Geometry: final body of the model. Coordinates: model frame, mm. Face numbers are marked on the shaded views. A direction names the side the tool comes from. Give positions to 0.01 mm unless a question says otherwise; leave off trailing zeros. Write each loop counter-clockwise with the first axis right and the second up, starting at its lowest first coordinate (ties: lowest second). Pieces come first, ordered by that corner, then holes. Notation, with made-up numbers: (-32, 50.5) -> (26, 50.5) arc R19 ccw to (26, 74.5) -> close; hole circle Ø4 at (68, 87). An arc over 180 degrees is marked (long way). Answer in a Markdown table with one row per item. Add a question column.
Item 1: Material intervals for probe 1 along Z at (x, y) = (61.5, 4.3); probe 2 along Z at (x, y) = (16, 7.8); probe 3 along X at (y, z) = (7.85, 12.5), sorted ascending. Write a range as from..to.
Item 2: Access query for the marked faces 1, 2 and 3. Directions: +Z, -Z, +X, -X, +Y, -Y. A direction counts if a zero-diameter tool reaches every point of the face in a straight line with its end or side. Return the directions, or none.
Item 3: Section query D-D on x = 61.5. State how many separate pieces and enclosed holes the cut face has, plus the area to 3 significant figures.
Item 4: Section query C-C on z = -4. Output: boundary loops of the cut face in (x, y).
Item 5: First-contact query: P1, Ø2.5, axis at x = 61.5, z = 4, coming from the +Y side; P2, Ø1.8, axis at x = 61.5, z = -4, coming from the +Y side; P3, Ø6, axis at y = 2.5, z = -12, coming from the +X side; P4, Ø3, axis at x = 45, y = 5, coming from the +Z side. Flat tips, straight axial feed; report the tip coordinate or a pass-through.
Item 6: Section query A-A on x = 16. Output: boundary loops of the cut face in (y, z), plus the area to 3 significant figures.
Item 7: Section query B-B on y = 8.75. Output: boundary loops of the cut face in (x, z), plus the area to 3 significant figures.
Autodesk Inventor part; units mm, degrees
ref_plane "YZ Plane" through (0, 0, 0) normal (1, 0, 0) x (0, 1, 0)
ref_plane "XZ Plane" through (0, 0, 0) normal (0, 1, 0) x (-1, 0, 0)
ref_plane "XY Plane" through (0, 0, 0) normal (0, 0, 1) x (1, 0, 0)
sketch "Sketch1" plane through (0, 0, 0) normal (0, 1, 0) x (-1, 0, 0)
  line L0 (-16, 12.5) -> (16, 12.5) construction
  line L1 (16, 12.5) -> (16, -12.5) construction
  line L2 (16, -12.5) -> (-16, -12.5) construction
  line L3 (-16, -12.5) -> (-16, 12.5) construction
  line L4 (-16, 12.5) -> (16, -12.5) construction
  line L5 (16, 12.5) -> (-16, -12.5) construction
  circle A0 centre (16, 12.5) radius 1.65
  circle A1 centre (16, -12.5) radius 1.65
  circle A2 centre (-16, -12.5) radius 1.65
  circle A3 centre (-16, 12.5) radius 1.65
  line L6 (-25, 17) -> (25, 17)
  line L7 (25, 17) -> (25, -17)
  line L8 (25, -17) -> (-25, -17)
  line L9 (-25, -17) -> (-25, 17)
  line L10 (-25, 17) -> (25, -17) construction
  line L11 (25, 17) -> (-25, -17) construction
  point P0 (0, 0)
  dimension "d0" = 32
  dimension "d1" = 25
  dimension "d2" = 3.3
  dimension "d3" = 3.3
  dimension "d4" = 3.3
  dimension "d5" = 3.3
  dimension "d6" = 50
  dimension "d7" = 34
extrude "Extrusion1" add sketch "Sketch1" along normal blind 10
sketch "Sketch2" plane through (0, 10, 0) normal (0, 1, 0) x (1, 0, 0)
  line L0 (-24, -7.5) -> (-12, -7.5)
  line L1 (-12, -7.5) -> (-12, 7.5)
  line L2 (-12, 7.5) -> (-24, 7.5)
  line L3 (-24, 7.5) -> (-24, -7.5)
  line L4 (-24, -7.5) -> (-12, 7.5) construction
  line L5 (-12, -7.5) -> (-24, 7.5) construction
  circle A0 centre (-16, -12.5) radius 1.65
  circle A1 centre (-16, -12.5) radius 3 construction
  point P0 (0, 0)
  point P1 (-18, 0)
  dimension "d10" = 18
  dimension "d11" = 15
  dimension "d12" = 6
  dimension "d13" = 12
extrude "Extrusion2" [suppressed]
sketch "Sketch5" plane through (0, 0, 0) normal (0, 0, 1) x (1, 0, 0)
  line L0 (25, 10) -> (-25, 10)
  line L1 (-21.2587, 10) -> (-11, 10)
  line L2 (-11, 10) -> (-11, 19.7515)
  line L3 (-11, 19.7515) -> (-17.6064, 31.6553)
  line L4 (-17.6064, 31.6553) -> (-28.0988, 25.8321)
  line L5 (-28.0988, 25.8321) -> (-21.2587, 13.5072)
  line L6 (-21.2587, 13.5072) -> (-21.2587, 10)
  circle A0 centre (-18, 20) radius 2.6308
  line L7 (-25, 0) -> (-25, 10)
  point P0 (0, 0)
  dimension "d22" = 7
  dimension "d23" = 10
  dimension "d24" = 7
  dimension "d26" = 6
  dimension "d27" = 6
  dimension "d28" = 10
extrude "Extrusion4" [suppressed]
sketch "Sketch6" plane through (-17.6064, 27.6553, 6) normal (0.8744, 0.4853, 0) x (0, 0, -1)
  circle A0 centre (3, -3) radius 1.1
  line L0 (12, 0) -> (0, 0)
  line L1 (0, -13.6141) -> (0, 0)
  line L2 (6, 0) -> (6, -13.6141) construction
  line L3 (12, -13.6141) -> (0, -13.6141)
  circle A1 centre (9, -3) radius 1.1
  point P0 (6, -32.7246)
  dimension "d31" = 3
  dimension "d32" = 3
  dimension "d38" = 2.2
extrude "Extrusion5" [suppressed]
sketch "Sketch7" plane through (0, 0, 6) normal (0, 0, 1) x (1, 0, 0)
  line L0 (-28.2228, 33.3896) -> (-18.3568, 15.6125)
  line L1 (-18.3568, 15.6125) -> (-17.4824, 16.0978)
  line L2 (-17.4824, 16.0978) -> (-27.3485, 33.8749)
  line L3 (-27.3485, 33.8749) -> (-28.2228, 33.3896)
  line L4 (-17.6064, 27.6553) -> (-28.0988, 21.8321)
  line L5 (-28.2228, 33.3896) -> (-17.4824, 16.0978) construction
  line L6 (-18.3568, 15.6125) -> (-27.3485, 33.8749) construction
  point P0 (0, 0)
  point P1 (-22.8526, 24.7437)
  dimension "d35" = 1
extrude "Extrusion6" [suppressed]
sketch "Sketch8" plane through (-21.2587, 9.5072, -6) normal (-0.8744, -0.4853, 0) x (0, 0, 1)
  circle A0 centre (9, 11.0958) radius 1.1
  circle A1 centre (9, 11.0958) radius 1.65
  circle A2 centre (3, 11.0958) radius 1.1
  circle A3 centre (3, 11.0958) radius 1.65
  point P0 (6, -18.6288)
  dimension "d39" = 3.3
  dimension "d40" = 3.3
extrude "Extrusion7" [suppressed]
fillet "Fillet1" [suppressed]
chamfer "Chamfer1" [suppressed]
sketch "Sketch9" plane through (0, 10, 0) normal (0, 1, 0) x (1, 0, 0)
  circle A0 centre (-16, 12.5) radius 1.65
  circle A1 centre (-16, 12.5) radius 3
  circle A2 centre (16, 12.5) radius 1.65
  circle A3 centre (16, 12.5) radius 3
  circle A4 centre (16, -12.5) radius 1.65
  circle A5 centre (16, -12.5) radius 3
  circle A6 centre (-16, -12.5) radius 1.65
  circle A7 centre (-16, -12.5) radius 3
  point P0 (0, 0)
  dimension "d47" = 6
  dimension "d48" = 6
  dimension "d49" = 6
  dimension "d50" = 6
extrude "Extrusion8" cut sketch "Sketch9" against normal blind 4 contours A0 | A1 | A3 | A5 | A7
fillet "Fillet2" radius 2 4 edges at (25, 5, 17) (25, 5, -17) (-25, 5, 17) (-25, 5, -17)
sketch "Sketch11" plane through (0, 0, 0) normal (0, 0, 1) x (1, 0, 0)
  line L0 (25, 10) -> (-25, 10)
  line L1 (25, 10) -> (65, 10)
  line L2 (65, 10) -> (65, 0)
  line L3 (65, 0) -> (25, 0)
  line L4 (25, 0) -> (25, 10)
  point P0 (0, 0)
  dimension "d54" = 40
  dimension "d55" = 10
extrude "Extrusion9" add sketch "Sketch11" along normal mid plane 15
sketch "Sketch12" plane through (0, 0, -7.5) normal (0, 0, -1) x (-1, 0, 0)
  line L0 (-65, 10) -> (-65, 0)
  line L1 (-65, 5) -> (-56.5, 5) construction
  circle A0 centre (-56.5, 5) radius 2.55
  line L2 (-67.1062, 5.5) -> (-57.7546, 5.5)
  line L3 (-57.7546, 5.5) -> (-57.7546, 4.5)
  line L4 (-57.7546, 4.5) -> (-67.1062, 4.5)
  line L5 (-67.1062, 4.5) -> (-67.1062, 5.5)
  line L6 (-67.1062, 5.5) -> (-57.7546, 4.5) construction
  line L7 (-57.7546, 5.5) -> (-67.1062, 4.5) construction
  point P0 (0, 0)
  point P1 (-62.4304, 5)
  point P2 (-59.0005, 4.5)
  point P3 (-59.0005, 5.5)
  dimension "d58" = 5.1
  dimension "d59" = 8.5
  dimension "d67" = 1
extrude "Extrusion10" cut sketch "Sketch12" against normal blind 15
sketch "Sketch13" plane through (0, 10, 0) normal (0, 1, 0) x (1, 0, 0)
  circle A0 centre (61.5, 4) radius 1.1
  line L0 (25, 7.5) -> (65, 7.5)
  line L1 (65, 7.5) -> (65, -7.5)
  line L2 (65, 7.5) -> (65, -7.5)
  line L3 (65, 0) -> (0, 0) construction
  circle A1 centre (61.5, -4) radius 1.1
  dimension "d62" = 3.5
  dimension "d63" = 3.5
  dimension "d64" = 2.2
extrude "Extrusion11" cut sketch "Sketch13" against normal blind 10.25
sketch "Sketch14" plane through (25, 0, 7.5) normal (0, -1, 0) x (1, 0, 0)
  circle A0 centre (36.5, -3.5) radius 1.1
  circle A1 centre (36.5, -3.5) radius 1.6
  circle A2 centre (36.5, -11.5) radius 1.1
  circle A3 centre (36.5, -11.5) radius 1.6
  point P0 (-25, -7.5)
  dimension "d68" = 3.2
  dimension "d69" = 3.2
extrude "Extrusion12" cut sketch "Sketch14" against normal blind 4 contours A0 | A1 | A2 | A3
fillet "Fillet3" radius 2 4 edges at (65, 7.75, -7.5) (65, 2.25, -7.5) (65, 2.25, 7.5) (65, 7.75, 7.5)
fillet "Fillet4" radius 2 2 edges at (25, 5, -7.5) (25, 5, 7.5)
equation "\"d3\" = d2"
equation "\"d4\" = d2"
equation "\"d5\" = d2"
equation "\"d48\" = d47"
equation "\"d49\" = d47"
equation "\"d50\" = d47"
equation "\"d69\" = d68"
properties part number "Puller"
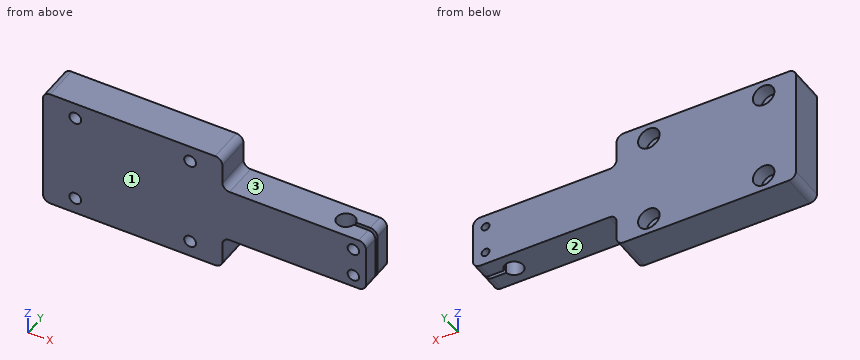
Findings below:
| question | item | result |
|---|---|---|
| 1 | probe 1 | z = -7.5..-5.1, -2.9..2.9, 5.1..7.5 |
| 1 | probe 2 | z = -17..-15.5, -9.5..9.5, 15.5..17 |
| 1 | probe 3 | x = -25..-19, -13..13, 19..25 |
| 2 | face 1 | +Z, -Z, +X, -X, -Y |
| 2 | face 2 | -Z, +X, +Y, -Y |
| 2 | face 3 | +Z, +X, +Y, -Y |
| 3 | separate pieces | 6 |
| 3 | enclosed holes | 0 |
| 3 | area | 87.4 mm^2 |
| 4 | outline | (-25, 0) -> (59.9, 0) -> (59.9, 4) -> (60.4, 4) -> (60.4, 4.5) -> (59, 4.5) arc R2.55 cw (long way) to (59, 5.5) -> (60.4, 5.5) -> (60.4, 10) -> (-25, 10) -> close; (62.6, 4) -> (63.1, 4) -> (63.1, 0) -> (65, 0) -> (65, 4.5) -> (62.6, 4.5) -> close; (62.6, 5.5) -> (65, 5.5) -> (65, 10) -> (62.6, 10) -> close |
| 5 | P1 | stops at y = 10 |
| 5 | P2 | passes through |
| 5 | P3 | stops at x = 25.06 |
| 5 | P4 | stops at z = 7.5 |
| 6 | outline | (0, -17) -> (10, -17) -> (10, -15.5) -> (6, -15.5) -> (6, -14.15) -> (0, -14.15) -> close; (0, -10.85) -> (6, -10.85) -> (6, -9.5) -> (10, -9.5) -> (10, 9.5) -> (6, 9.5) -> (6, 10.85) -> (0, 10.85) -> close; (0, 14.15) -> (6, 14.15) -> (6, 15.5) -> (10, 15.5) -> (10, 17) -> (0, 17) -> close |
| 6 | area | 252 mm^2 |
| 7 | outline | (-25, -15) arc R2 ccw to (-23, -17) -> (23, -17) arc R2 ccw to (25, -15) -> (25, -9.5) arc R2 cw to (27, -7.5) -> (63, -7.5) arc R2 ccw to (65, -5.5) -> (65, 5.5) arc R2 ccw to (63, 7.5) -> (27, 7.5) arc R2 cw to (25, 9.5) -> (25, 15) arc R2 ccw to (23, 17) -> (-23, 17) arc R2 ccw to (-25, 15) -> close; hole circle Ø6 at (-16, -12.5); hole circle Ø6 at (-16, 12.5); hole circle Ø6 at (16, -12.5); hole circle Ø6 at (16, 12.5); hole circle Ø2.2 at (61.5, -4); hole circle Ø2.2 at (61.5, 4) |
| 7 | area | 2,180 mm^2 |
